from build123d import *

# Parameters (mm, degrees)
BOSS_EXTRUDE1_DEPTH     = 2
CONVERT_SOLID1_DEPTH    = 0.5
EDGE_FLANGE1_DEPTH      = 440
EDGE_FLANGE1_BEND_DEPTH = 440
SKETCH12_R              = 2.25
CUT_EXTRUDE1_DEPTH      = 1.5


# Read off the part's stored shape, not the designer's step: Convert-Solid1
# Sheet-metal steps are written as plain solids
with BuildPart() as part:
    # Model → Boss-Extrude1 (new body)
    with BuildSketch(Plane.XY):
        with BuildLine():
            Line((221.66, -19.508939372), (221.66, -21.75))
            ThreePointArc((221.66, -21.75), (221.733223305, -21.926776695), (221.91, -22))
            Line((221.91, -22), (241.25, -22))
            ThreePointArc((241.25, -22), (241.426776695, -21.926776695), (241.5, -21.75))
            Line((241.5, -21.75), (241.5, 21.75))
            Line((241.5, 21.75), (241.500000169, 22.249478564))
            Line((241.500000169, 22.249478564), (241.500000169, 65.749478564))
            ThreePointArc((241.500000169, 65.749478564), (241.426776865, 65.926255259), (241.250000169, 65.999478564))
            Line((241.250000169, 65.999478564), (221.910000169, 65.999478564))
            ThreePointArc((221.910000169, 65.999478564), (221.733223474, 65.926255259), (221.660000169, 65.749478564))
            Line((221.660000169, 65.749478564), (221.660000169, 63.508417937))
            ThreePointArc((221.660000169, 63.508417937), (221.580000169, 63.428417937), (221.500000169, 63.508417937))
            Line((221.500000169, 63.508417937), (221.500000169, 63.928417937))
            Line((221.500000169, 63.928417937), (-221.499999831, 63.928417937))
            Line((-221.499999831, 63.928417937), (-221.499999831, 63.508417937))
            ThreePointArc((-221.499999831, 63.508417937), (-221.579999831, 63.428417937), (-221.659999831, 63.508417937))
            Line((-221.659999831, 63.508417937), (-221.659999831, 65.749478564))
            ThreePointArc((-221.659999831, 65.749478564), (-221.733223135, 65.926255259), (-221.909999831, 65.999478564))
            Line((-221.909999831, 65.999478564), (-241.249999831, 65.999478564))
            ThreePointArc((-241.249999831, 65.999478564), (-241.426776526, 65.926255259), (-241.499999831, 65.749478564))
            Line((-241.499999831, 65.749478564), (-241.499999831, 22.249478564))
            Line((-241.499999831, 22.249478564), (-241.5, 21.75))
            Line((-241.5, 21.75), (-241.5, -21.75))
            ThreePointArc((-241.5, -21.75), (-241.426776695, -21.926776695), (-241.25, -22))
            Line((-241.25, -22), (-221.91, -22))
            ThreePointArc((-221.91, -22), (-221.733223305, -21.926776695), (-221.66, -21.75))
            Line((-221.66, -21.75), (-221.66, -19.508939372))
            ThreePointArc((-221.66, -19.508939372), (-221.58, -19.428939372), (-221.5, -19.508939372))
            Line((-221.5, -19.508939372), (-221.5, -19.928939372))
            Line((-221.5, -19.928939372), (221.5, -19.928939372))
            Line((221.5, -19.928939372), (221.5, -19.508939372))
            ThreePointArc((221.5, -19.508939372), (221.58, -19.428939372), (221.66, -19.508939372))
        make_face()
        with BuildLine():
            Line((-231.25, -19.5), (-234.75, -19.5))
            ThreePointArc((-234.75, -19.5), (-238, -16.25), (-234.75, -13))
            Line((-234.75, -13), (-231.25, -13))
            ThreePointArc((-231.25, -13), (-228, -16.25), (-231.25, -19.5))
        make_face(mode=Mode.SUBTRACT)
        with BuildLine():
            Line((231.25, -13), (234.75, -13))
            ThreePointArc((234.75, -13), (238, -16.25), (234.75, -19.5))
            Line((234.75, -19.5), (231.25, -19.5))
            ThreePointArc((231.25, -19.5), (228, -16.25), (231.25, -13))
        make_face(mode=Mode.SUBTRACT)
        with BuildLine():
            Line((-231.249999831, 56.999478564), (-234.749999831, 56.999478564))
            ThreePointArc((-234.749999831, 56.999478564), (-237.999999831, 60.249478564), (-234.749999831, 63.499478564))
            Line((-234.749999831, 63.499478564), (-231.249999831, 63.499478564))
            ThreePointArc((-231.249999831, 63.499478564), (-227.999999831, 60.249478564), (-231.249999831, 56.999478564))
        make_face(mode=Mode.SUBTRACT)
        with BuildLine():
            Line((234.750000169, 56.999478564), (231.250000169, 56.999478564))
            ThreePointArc((231.250000169, 56.999478564), (228.000000169, 60.249478564), (231.250000169, 63.499478564))
            Line((231.250000169, 63.499478564), (234.750000169, 63.499478564))
            ThreePointArc((234.750000169, 63.499478564), (238.000000169, 60.249478564), (234.750000169, 56.999478564))
        make_face(mode=Mode.SUBTRACT)
    extrude(amount=BOSS_EXTRUDE1_DEPTH)

    # Convert-Solid1 outline → Convert-Solid1 (cut)
    with BuildSketch(Plane.XY):
        with BuildLine():
            Line((221.5, -19.928939372), (221.5, -19.508939372))
            ThreePointArc((221.5, -19.508939372), (221.58, -19.428939372), (221.66, -19.508939372))
            Line((221.66, -19.508939372), (221.66, -21.75))
            ThreePointArc((221.66, -21.75), (221.733223305, -21.926776695), (221.91, -22))
            Line((221.91, -22), (241.25, -22))
            ThreePointArc((241.25, -22), (241.426776695, -21.926776695), (241.5, -21.75))
            Line((241.5, -21.75), (241.5, 21.75))
            Line((241.5, 21.75), (241.500000169, 65.749478564))
            ThreePointArc((241.500000169, 65.749478564), (241.426776864, 65.926255259), (241.250000169, 65.999478564))
            Line((241.250000169, 65.999478564), (221.910000169, 65.999478564))
            ThreePointArc((221.910000169, 65.999478564), (221.733223474, 65.926255259), (221.660000169, 65.749478564))
            Line((221.660000169, 65.749478564), (221.660000169, 63.508417937))
            ThreePointArc((221.660000169, 63.508417937), (221.580000169, 63.428417937), (221.500000169, 63.508417937))
            Line((221.500000169, 63.508417937), (221.500000169, 63.928417937))
            Line((221.500000169, 63.928417937), (-221.499999831, 63.928417937))
            Line((-221.499999831, 63.928417937), (-221.499999831, 63.508417937))
            ThreePointArc((-221.499999831, 63.508417937), (-221.579999831, 63.428417937), (-221.659999831, 63.508417937))
            Line((-221.659999831, 63.508417937), (-221.659999831, 65.749478564))
            ThreePointArc((-221.659999831, 65.749478564), (-221.733223135, 65.926255259), (-221.909999831, 65.999478564))
            Line((-221.909999831, 65.999478564), (-241.249999831, 65.999478564))
            ThreePointArc((-241.249999831, 65.999478564), (-241.426776526, 65.926255259), (-241.499999831, 65.749478564))
            Line((-241.499999831, 65.749478564), (-241.499999831, 22.249478564))
            Line((-241.499999831, 22.249478564), (-241.5, -21.75))
            ThreePointArc((-241.5, -21.75), (-241.426776695, -21.926776695), (-241.25, -22))
            Line((-241.25, -22), (-221.91, -22))
            ThreePointArc((-221.91, -22), (-221.733223305, -21.926776695), (-221.66, -21.75))
            Line((-221.66, -21.75), (-221.66, -19.508939372))
            ThreePointArc((-221.66, -19.508939372), (-221.58, -19.428939372), (-221.5, -19.508939372))
            Line((-221.5, -19.508939372), (-221.5, -19.928939372))
            Line((-221.5, -19.928939372), (221.5, -19.928939372))
        make_face()
        with BuildLine():
            Line((-234.75, -13), (-231.25, -13))
            ThreePointArc((-231.25, -13), (-228, -16.25), (-231.25, -19.5))
            Line((-231.25, -19.5), (-234.75, -19.5))
            ThreePointArc((-234.75, -19.5), (-238, -16.25), (-234.75, -13))
        make_face(mode=Mode.SUBTRACT)
        with BuildLine():
            ThreePointArc((231.25, -19.5), (228, -16.25), (231.25, -13))
            Line((231.25, -13), (234.75, -13))
            ThreePointArc((234.75, -13), (238, -16.25), (234.75, -19.5))
            Line((234.75, -19.5), (231.25, -19.5))
        make_face(mode=Mode.SUBTRACT)
        with BuildLine():
            Line((-234.749999831, 63.499478564), (-231.249999831, 63.499478564))
            ThreePointArc((-231.249999831, 63.499478564), (-227.999999831, 60.249478564), (-231.249999831, 56.999478564))
            Line((-231.249999831, 56.999478564), (-234.749999831, 56.999478564))
            ThreePointArc((-234.749999831, 56.999478564), (-237.999999831, 60.249478564), (-234.749999831, 63.499478564))
        make_face(mode=Mode.SUBTRACT)
        with BuildLine():
            ThreePointArc((231.250000169, 56.999478564), (228.000000169, 60.249478564), (231.250000169, 63.499478564))
            Line((231.250000169, 63.499478564), (234.750000169, 63.499478564))
            ThreePointArc((234.750000169, 63.499478564), (238.000000169, 60.249478564), (234.750000169, 56.999478564))
            Line((234.750000169, 56.999478564), (231.250000169, 56.999478564))
        make_face(mode=Mode.SUBTRACT)
    extrude(amount=CONVERT_SOLID1_DEPTH, mode=Mode.SUBTRACT)

    # Edge-Flange1 section (across the edge) → Edge-Flange1 (add)
    with BuildSketch(Plane(origin=(-219.999999831, 65.428417937, 0.5), x_dir=(0, -1, 0), z_dir=(1, 0, 0))):
        with BuildLine():
            Line((-1.5, 1.5), (-1.5, 13.5))
            Line((-1.5, 13.5), (0, 13.5))
            Line((0, 13.5), (0, 1.5))
            ThreePointArc((0, 1.5), (0.439339828, 0.439339828), (1.5, 0))
            Line((1.5, 0), (1.5, -1.5))
            ThreePointArc((1.5, -1.5), (-0.621320344, -0.621320344), (-1.5, 1.5))
        make_face()
    extrude(amount=EDGE_FLANGE1_DEPTH)

    # Edge-Flange1 section 2 (across the edge) → Edge-Flange1 bend (add)
    with BuildSketch(Plane(origin=(220, -21.428939372, 0.5), x_dir=(0, 1, 0), z_dir=(-1, 0, 0))):
        with BuildLine():
            Line((-1.5, 1.5), (-1.5, 13.5))
            Line((-1.5, 13.5), (0, 13.5))
            Line((0, 13.5), (0, 1.5))
            ThreePointArc((0, 1.5), (0.439339828, 0.439339828), (1.5, 0))
            Line((1.5, 0), (1.5, -1.5))
            ThreePointArc((1.5, -1.5), (-0.621320344, -0.621320344), (-1.5, 1.5))
        make_face()
    extrude(amount=EDGE_FLANGE1_BEND_DEPTH)

    # Sketch12 → Cut-Extrude1 (cut)
    with BuildSketch(Plane.XY.offset(2)):
        with Locations((211.000000169, 57.937539282)):
            Circle(SKETCH12_R)
        with Locations((23.040000169, 57.937539282)):
            Circle(SKETCH12_R)
        with Locations((23.040000169, -13.938060718)):
            Circle(SKETCH12_R)
        with Locations((211.000000169, -13.938060718)):
            Circle(SKETCH12_R)
        with BuildLine():
            Line((34.420000169, 54.437539282), (199.620000169, 54.437539282))
            ThreePointArc((199.620000169, 54.437539282), (205.192001605, 52.129540718), (207.500000169, 46.557539282))
            Line((207.500000169, 46.557539282), (207.500000169, -2.558060718))
            ThreePointArc((207.500000169, -2.558060718), (205.192001605, -8.130062154), (199.620000169, -10.438060718))
            Line((199.620000169, -10.438060718), (34.420000169, -10.438060718))
            ThreePointArc((34.420000169, -10.438060718), (28.847998734, -8.130062154), (26.540000169, -2.558060718))
            Line((26.540000169, -2.558060718), (26.540000169, 46.557539282))
            ThreePointArc((26.540000169, 46.557539282), (28.847998734, 52.129540718), (34.420000169, 54.437539282))
        make_face()
    extrude(amount=-CUT_EXTRUDE1_DEPTH, mode=Mode.SUBTRACT)


solid = part.part
Model file for the job. Use its own axes, mm. A direction names the side the tool comes from. Give positions to 0.01 mm unless a question says otherwise; leave off trailing zeros. Loops run counter-clockwise (first coordinate to the right, second up) from the corner with the lowest first, then second, coordinate; pieces in that order, holes last.
Item 1: Drop flat-ended pins along their axis: P1, Ø8, axis at y = 49.5, z = -1.5, coming from the -X side; P2, Ø12, axis at x = -34.5, y = 11.5, coming from the -Z side; P3, Ø0.8, axis at x = -221, z = 1.5, coming from the +Y side; P4, Ø1.2, axis at x = -233.5, z = 1, coming from the +Y side. Give the stop position or say it passes through.
Check values:
P1: stops at x = -241.5
P2: stops at z = 0.5
P3: stops at y = 63.93
P4: stops at y = 66
Item 2: Drill centre lines: line 1 along Y through (x, z) = (23.04, 1.2); line 2 along Y through (x, z) = (-159, -11.5); line 3 along Y through (x, z) = (23.04, 1.7). Where is each one in solid material? Low to high.
Check values:
line 1: y = -21.97 to -16.19, -11.69 to 55.69, 60.19 to 65.97
line 2: y = -22.93 to -21.43, 65.43 to 66.93
line 3: y = -21.24 to -16.19, -11.69 to 55.69, 60.19 to 65.24
Item 3: Mould opens along Y. For faces 1 (the face through (3, -22.929, -7)), 2 (the face through (-3, 66.928, -7)), 3 (the face through (205.13, 52.19, 1.26)), 4 (the face through (-3, 65.428, -7)) say: +Y half, -Y half, draft (parallel to the pull), parting line (faces both ways), or undercut.
Check values:
face 1: -Y half
face 2: +Y half
face 3: undercut
face 4: undercut
Item 4: Slice it at A-A (z = -9.25). Write the cut outline in (x, y).
Check values:
outline: (-220, -22.93) - (220, -22.93) - (220, -21.43) - (-220, -21.43) - close; (-220, 65.43) - (220, 65.43) - (220, 66.93) - (-220, 66.93) - close
Item 5: Slice it at B-B (x = 76.5). Write the cut outline in (y, z), plus the area to 3 significant figures.
Check values:
outline: (-22.93, -13) - (-21.43, -13) - (-21.43, -1) arc R1.5 cw to (-19.93, 0.5) - (-10.44, 0.5) - (-10.44, 2) - (-19.93, 2) arc R3 ccw to (-22.93, -1) - close; (54.44, 0.5) - (63.93, 0.5) arc R1.5 cw to (65.43, -1) - (65.43, -13) - (66.93, -13) - (66.93, -1) arc R3 ccw to (63.93, 2) - (54.44, 2) - close
area: 75.1 mm2
Item 6: Slice it at D-D (x = -146). Write the cut outline in (y, z), plus the area to 3 significant figures.
Check values:
outline: (-22.93, -13) - (-21.43, -13) - (-21.43, -1) arc R1.5 cw to (-19.93, 0.5) - (63.93, 0.5) arc R1.5 cw to (65.43, -1) - (65.43, -13) - (66.93, -13) - (66.93, -1) arc R3 ccw to (63.93, 2) - (-19.93, 2) arc R3 ccw to (-22.93, -1) - close
area: 172 mm2
Item 7: Which spindle directions (+Z, -Z, +X, -X, +Y, -Y) get a long thin tool onto all of the face, cutting with end or side? Do faces 5 (the face through (28.79, 52.07, 1.26)), 6 (the face through (3, -21.429, -7)), 7 (the face through (-57, 23, 2)). Say none if no direction does.
Check values:
face 5: +Z, -Z
face 6: -Z, +X, -X
face 7: +Z, +X, -X, +Y, -Y
Item 8: Slice it at C-C (y = 35.5). Write the cut outline in (x, z), plus the area to 3 significant figures.
Check values:
outline: (-241.5, 0.5) - (26.54, 0.5) - (26.54, 2) - (-241.5, 2) - close; (207.5, 0.5) - (241.5, 0.5) - (241.5, 2) - (207.5, 2) - close
area: 453 mm2
